Model file for the job. Use its own axes, mm. A direction names the side the tool comes from. Round coordinates to 2 decimals unless told otherwise and drop trailing zeros. Order: outer loops, then holes, each group sorted by start corner. A loop starts at its lowest first (then second) coordinate and runs counter-clockwise, first axis right, second up. Notation, with made-up numbers: M 14.5,29 L 65.5,29 A14 ccw 65.5,50 Z; hole C -20,80.25 d8. An arc over 180 degrees is marked long. Return JSON: item names as keys, results as strings. Group by question number.
Item 1: Slice it at A-A on z = 30. Write the cut outline in (x, y), then the cut area to 3 significant figures.
Item 2: Which spindle directions (+Z, -Z, +X, -X, +Y, -Y) get a long thin tool onto all of the face, cutting with end or side? Do faces 1 (the face through (0, 0, 19)), 2 (the face through (0, 6, 16)), 3 (the face through (0, 16, 6)), 4 (the face through (0, 37, 5)). Say none if no direction does.
Item 3: Pull direction X, two halves, no side cores. Call faces 5 (the face through (0, 3, 37)), 6 (the face through (-0.358, 52.727, 2.465)), 7 (the face through (0.121, 2.465, 27.253)), 8 (the face through (-7, 16, 12)): pulls with the +X half, pulls with the -X half, needs draft (parallel to the pull), parting line crosses it, or undercut.
Item 4: Pin check, flat tips, straight feed: pin 1 Ø7 at (x, z) = (0.5, 24) entering from +Y; pin 2 Ø6 at (x, z) = (-1.5, 17) entering from +Y; pin 3 Ø6.5 at (x, y) = (0, 50) entering from +Z. Stop position of each tip, or through.
Item 5: Probe line 1 along Y through (x, z) = (0, 2); line 2 along Z through (x, y) = (3.25, 12); line 3 along X through (y, z) = (1.9, 30). List the from-to ranges inside material, lowest first.
Item 6: Slice it at D-D on z = 19. Write the cut outline in (x, y).
Item 7: Slice it at C-C on x = -4.75. Write the cut outline in (y, z), then the cut area to 3 significant figures.
from build123d import *

# Parameters (mm, degrees)
BOSS_EXTRUDE1_DEPTH      = 7
BOSS_EXTRUDE1_DEPTH_BACK = 7
SKETCH2_R                = 2.75
CUT_EXTRUDE1_DEPTH       = 5
SKETCH3_R                = 2.75
CUT_EXTRUDE2_DEPTH       = 5
SKETCH4_R                = 2.75
CUT_EXTRUDE3_DEPTH       = 5


with BuildPart() as part:
    # Sketch1 → Boss-Extrude1 (new, two sides: drawn at the far end of the back side and taken through both)
    with BuildSketch(Plane(origin=(0, 0, 0), x_dir=(0, 0, -1), z_dir=(1, 0, 0)).offset(-BOSS_EXTRUDE1_DEPTH_BACK)):
        with BuildLine():
            Line((-36, 0), (-1, 0))
            ThreePointArc((-1, 0), (-0.292893219, 0.292893219), (0, 1))
            Line((0, 1), (0, 56))
            ThreePointArc((0, 56), (-0.292893219, 56.707106781), (-1, 57))
            Line((-1, 57), (-4, 57))
            ThreePointArc((-4, 57), (-4.707106781, 56.707106781), (-5, 56))
            Line((-5, 56), (-5, 17.414213562))
            ThreePointArc((-5, 17.414213562), (-5.076120467, 17.03153013), (-5.292893219, 16.707106781))
            Line((-5.292893219, 16.707106781), (-7.121957509, 14.878042491))
            ThreePointArc((-7.121957509, 14.878042491), (-7.866746852, 14.585859512), (-8.587416263, 14.93330398))
            ThreePointArc((-8.587416263, 14.93330398), (-10.519537583, 16.249497739), (-12.851234525, 16.418755456))
            ThreePointArc((-12.851234525, 16.418755456), (-13.048766707, 16.283360738), (-13.084263382, 16.046526031))
            Line((-13.084263382, 16.046526031), (-12.616293745, 14.300039569))
            ThreePointArc((-12.616293745, 14.300039569), (-12.492491512, 14.127781044), (-12.285701536, 14.080474617))
            ThreePointArc((-12.285701536, 14.080474617), (-10.515075746, 10.515075773), (-14.080474622, 12.285701498))
            ThreePointArc((-14.080474622, 12.285701498), (-14.127781033, 12.492491496), (-14.300039569, 12.616293745))
            Line((-14.300039569, 12.616293745), (-16.046526031, 13.084263382))
            ThreePointArc((-16.046526031, 13.084263382), (-16.283360688, 13.048766739), (-16.418755434, 12.851234641))
            ThreePointArc((-16.418755434, 12.851234641), (-16.249497766, 10.51953766), (-14.933304014, 8.587416292))
            ThreePointArc((-14.933304014, 8.587416292), (-14.585859513, 7.866746874), (-14.878042491, 7.121957509))
            Line((-14.878042491, 7.121957509), (-16.707106781, 5.292893219))
            ThreePointArc((-16.707106781, 5.292893219), (-17.03153013, 5.076120467), (-17.414213562, 5))
            Line((-17.414213562, 5), (-36, 5))
            ThreePointArc((-36, 5), (-36.707106781, 4.707106781), (-37, 4))
            Line((-37, 4), (-37, 1))
            ThreePointArc((-37, 1), (-36.707106781, 0.292893219), (-36, 0))
        make_face()
    extrude(amount=BOSS_EXTRUDE1_DEPTH + BOSS_EXTRUDE1_DEPTH_BACK)

    # Sketch2 → Cut-Extrude1 (cut)
    with BuildSketch(Plane.XY):
        with Locations((0, 30)):
            Circle(SKETCH2_R)
    extrude(amount=CUT_EXTRUDE1_DEPTH, mode=Mode.SUBTRACT)

    # Sketch3 → Cut-Extrude2 (cut)
    with BuildSketch(Plane.XY):
        with Locations((0, 50)):
            Circle(SKETCH3_R)
    extrude(amount=CUT_EXTRUDE2_DEPTH, mode=Mode.SUBTRACT)

    # Sketch4 → Cut-Extrude3 (cut)
    with BuildSketch(Plane(origin=(0, 0, 0), x_dir=(1, 0, 0), z_dir=(0, 1, 0))):
        with Locations(Location((0, -30, 0), (0, 0, 270))):
            Circle(SKETCH4_R)
    extrude(amount=CUT_EXTRUDE3_DEPTH, mode=Mode.SUBTRACT)


solid = part.part
Output values:
{
 "1": {"outline": "M -7,0 L -2.75,0 L -2.75,5 L -7,5 Z; M 2.75,0 L 7,0 L 7,5 L 2.75,5 Z", "area": "42.5 mm²"},
 "2": {"face 1": "+Z, -Z, +X, -X, -Y", "face 2": "+Z, +X, -X", "face 3": "+X, -X, +Y", "face 4": "+Z, +X, -X, +Y"},
 "3": {"face 5": "needs draft", "face 6": "undercut", "face 7": "undercut", "face 8": "pulls with the -X half"},
 "4": {"pin 1": "y = 5", "pin 2": "y = 13.09", "pin 3": "z = 5"},
 "5": {"line 1": "0 to 27.25, 32.75 to 47.25, 52.75 to 57", "line 2": "0 to 9.9, 14.1 to 16.5", "line 3": "-7 to -2.75, 2.75 to 7"},
 "6": {"outline": "M -7,0 L 7,0 L 7,5 L -7,5 Z"},
 "7": {"outline": "M 0,1 A1 ccw 1,0 L 56,0 A1 ccw 57,1 L 57,4 A1 ccw 56,5 L 17.41,5 A1 cw 16.71,5.29 L 14.88,7.12 A1 cw 14.93,8.59 A4.5 ccw 16.42,12.85 A0.3 ccw 16.05,13.08 L 14.3,12.62 A0.3 ccw 14.08,12.29 A2.1 cw long 12.29,14.08 A0.3 ccw 12.62,14.3 L 13.08,16.05 A0.3 ccw 12.85,16.42 A4.5 ccw 8.59,14.93 A1 cw 7.12,14.88 L 5.29,16.71 A1 cw 5,17.41 L 5,36 A1 ccw 4,37 L 1,37 A1 ccw 0,36 Z", "area": "539 mm²"}
}
